Source: three-view drawing plus pictorial views. Frame: mm from the lowest corner of the part. A direction names the side the tool comes from. Give positions to 0.01 mm unless a question says otherwise; leave off trailing zeros. Write each loop counter-clockwise with the first axis right and the second up, starting at its lowest first coordinate (ties: lowest second). Pieces come first, ordered by that corner, then holes.
Q1. Cut plane D-D on z = 206. Return the cut outline in (x, y).
Q2. Cut plane C-C on y = 434.5. Return the cut outline in (x, z), plus the area to 3 significant figures.
Q3. Pin query (flat end, axial travel): pin 1 (8 mm diameter, centred on x = 238.5, y = 274.5, fed in from -Z); pin 2 (1 mm diameter, centred on y = 226.5, z = 336, fed in from -X); pin 3 (22 mm diameter, centred on x = 274, y = 96.5, fed in from +Z). Return the tip coordinate at first contact, or that it passes through.
Q4. Cut plane B-B on z = 55. Return the cut outline in (x, y) (1 decimal), plus the area to 3 significant figures.
Q5. Line query: L1, parallel to Y at x = 101, z = 149; L2, parallel to Z at x = 160, y = 210 (1 decimal); L3, parallel to X at y = 208, z = 375. Output: solid intervals per line, ascending.
Q6. Reachability of the marked faces 4, 5 and 6 from +Z, -Z, +X, -X, +Y, -Y: full face, straight path, thin tool, end or side. Return the list, or none.
Q7. Draft query along Z for the marked faces 1, 2 and 3. Return one class per face: pulls with the +Z half, pulls with the -Z half, needs draft (parallel to the pull), parting line crosses it, or undercut.
Q8. Cut plane A-A on z = 114. Return the cut outline in (x, y), plus the area to 3 significant figures.
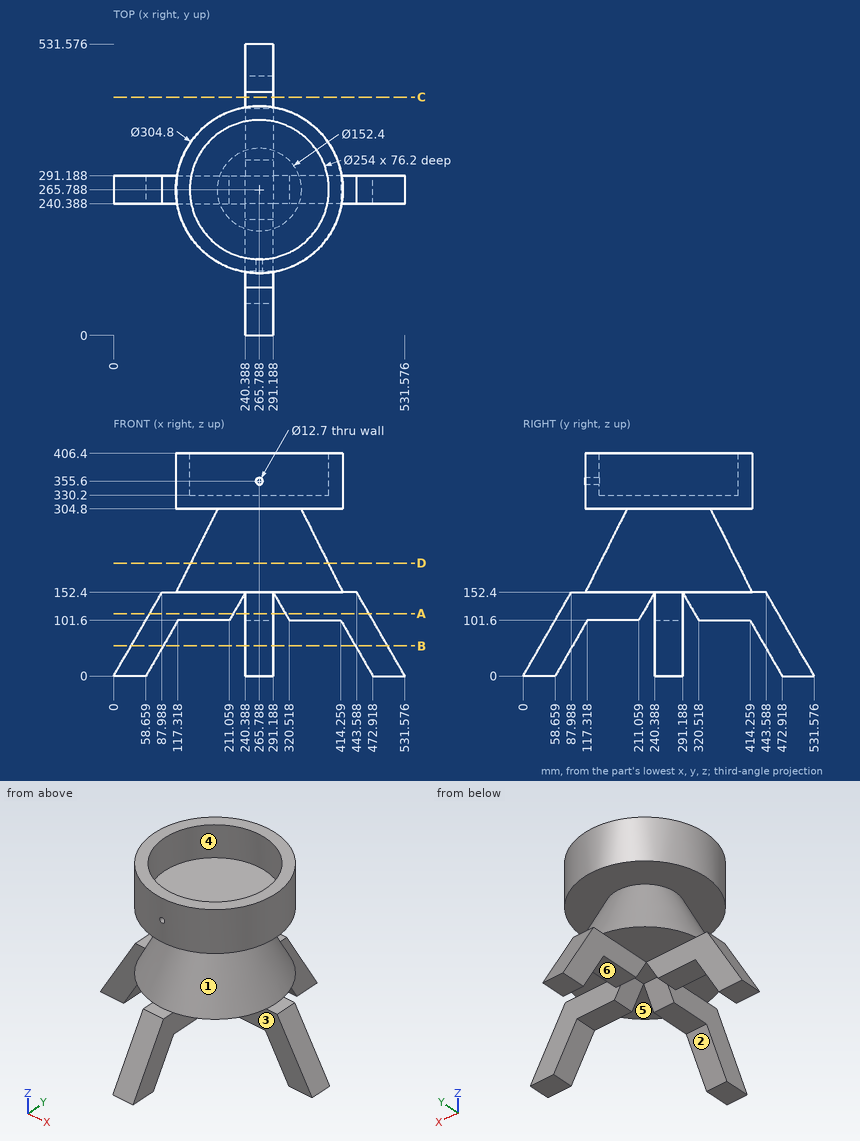
Data:
1. outline: circle Ø251.2 at (265.79, 265.79)
2. outline: (240.39, 66.54) - (291.19, 66.54) - (291.19, 152.4) - (240.39, 152.4) - close
2. area: 4,360 mm2
3. pin 1: stops at z = 142.2
3. pin 2: stops at x = 118.41
3. pin 3: stops at z = 152.4
4. outline: (31.8, 240.4) - (90.4, 240.4) - (90.4, 291.2) - (31.8, 291.2) - close; (240.4, 31.8) - (291.2, 31.8) - (291.2, 90.4) - (240.4, 90.4) - close; (240.4, 441.2) - (291.2, 441.2) - (291.2, 499.8) - (240.4, 499.8) - close; (441.2, 240.4) - (499.8, 240.4) - (499.8, 291.2) - (441.2, 291.2) - close
4. area: 11,900 mm2
5. L1: y = 240.39 to 291.19
5. L2: z = 152.4 to 218, 304.8 to 330.2
5. L3: x = 124.77 to 152.7, 378.88 to 406.81
6. face 4: +Z
6. face 5: -Z, +X, -Y
6. face 6: -Z, +X, -X
7. face 1: undercut
7. face 2: pulls with the -Z half
7. face 3: needs draft
8. outline: (65.82, 240.39) - (218.22, 240.39) - (218.22, 291.19) - (65.82, 291.19) - close; (240.39, 65.82) - (291.19, 65.82) - (291.19, 218.22) - (240.39, 218.22) - close; (240.39, 313.36) - (291.19, 313.36) - (291.19, 465.76) - (240.39, 465.76) - close; (313.36, 240.39) - (465.76, 240.39) - (465.76, 291.19) - (313.36, 291.19) - close
8. area: 31,000 mm2
